The model under review builds one solid part; all positions refer to its coordinate system, in mm. A direction names the side the tool comes from. Coordinates: 2 decimals unless noted, no trailing zeros. Loops run counter-clockwise (first coordinate to the right, second up) from the corner with the lowest first, then second, coordinate; pieces in that order, holes last. Notation, with made-up numbers: M 24.5,-19.75 L 80.5,-19.75 A17 ccw 80.5,-6.75 Z; hole C -32.75,34.5 d6. An arc over 180 degrees is marked long. Return JSON: item names as keys, results as strings.
```python
from build123d import *

# Parameters (mm, degrees)
SKETCH1_R           = 2.542419914
BOSS_EXTRUDE1_DEPTH = 3.999992


with BuildPart() as part:
    # Sketch1 → Boss-Extrude1 (new body)
    with BuildSketch(Plane(origin=(0, 0, 0), x_dir=(1, 0, 0), z_dir=(0, 1, 0))):
        with BuildLine():
            Line((-7.927115113, 2.735422797), (-7.212976361, 2.491621041))
            ThreePointArc((-7.212976361, 2.491621041), (-6.913293064, 2.224424018), (-6.895509083, 1.823315483))
            ThreePointArc((-6.895509083, 1.823315483), (-6.953671189, 1.587130072), (-7.003745952, 1.349098778))
            ThreePointArc((-7.003745952, 1.349098778), (-7.193803236, 0.995428655), (-7.579741, 0.884720165))
            Line((-7.579741, 0.884720165), (-8.3289394, 0.974915565))
            ThreePointArc((-8.3289394, 0.974915565), (-9.212212433, 0.780173764), (-9.9866958, 0.3129788))
            Line((-9.9866958, 0.3129788), (-9.9866958, -0.3129788))
            ThreePointArc((-9.9866958, -0.3129788), (-9.212212433, -0.780173764), (-8.3289394, -0.974915565))
            Line((-8.3289394, -0.974915565), (-7.579741, -0.884720165))
            ThreePointArc((-7.579741, -0.884720165), (-7.193803236, -0.995428655), (-7.003745952, -1.349098778))
            ThreePointArc((-7.003745952, -1.349098778), (-6.953671189, -1.587130072), (-6.895509083, -1.823315483))
            ThreePointArc((-6.895509083, -1.823315483), (-6.913293064, -2.224424018), (-7.212976361, -2.491621041))
            Line((-7.212976361, -2.491621041), (-7.927115113, -2.735422797))
            ThreePointArc((-7.927115113, -2.735422797), (-8.638421316, -3.294116903), (-9.133498421, -4.05108076))
            Line((-9.133498421, -4.05108076), (-8.861905597, -4.61504907))
            ThreePointArc((-8.861905597, -4.61504907), (-7.961411897, -4.699941449), (-7.081115091, -4.492159943))
            Line((-7.081115091, -4.492159943), (-6.445244975, -4.085831692))
            ThreePointArc((-6.445244975, -4.085831692), (-6.049492451, -4.018124475), (-5.724805039, -4.25430748))
            ThreePointArc((-5.724805039, -4.25430748), (-5.576411329, -4.44703964), (-5.421532073, -4.63459975))
            ThreePointArc((-5.421532073, -4.63459975), (-5.263520415, -5.003702234), (-5.417593292, -5.374466142))
            Line((-5.417593292, -5.374466142), (-5.955228458, -5.903977126))
            ThreePointArc((-5.955228458, -5.903977126), (-6.353684915, -6.715967318), (-6.471299665, -7.612774092))
            Line((-6.471299665, -7.612774092), (-5.981906306, -8.003052272))
            ThreePointArc((-5.981906306, -8.003052272), (-5.133756094, -7.688828089), (-4.430789095, -7.119676951))
            Line((-4.430789095, -7.119676951), (-4.034189136, -6.477694143))
            ThreePointArc((-4.034189136, -6.477694143), (-3.707005493, -6.244981464), (-3.311996278, -6.31689841))
            ThreePointArc((-3.311996278, -6.31689841), (-3.094674815, -6.426158468), (-2.873754145, -6.527944698))
            ThreePointArc((-2.873754145, -6.527944698), (-2.571242995, -6.791935856), (-2.54918943, -7.192832311))
            Line((-2.54918943, -7.192832311), (-2.80383577, -7.903176378))
            ThreePointArc((-2.80383577, -7.903176378), (-2.810523293, -8.807638039), (-2.527380645, -9.666664151))
            Line((-2.527380645, -9.666664151), (-1.917117109, -9.805952821))
            ThreePointArc((-1.917117109, -9.805952821), (-1.289296936, -9.154848028), (-0.902890978, -8.337054622))
            Line((-0.902890978, -8.337054622), (-0.824112663, -7.586569825))
            ThreePointArc((-0.824112663, -7.586569825), (-0.630300635, -7.234943284), (-0.243206036, -7.128350138))
            ThreePointArc((-0.243206036, -7.128350138), (0, -7.1324978), (0.243206036, -7.128350138))
            ThreePointArc((0.243206036, -7.128350138), (0.630300635, -7.234943284), (0.824112663, -7.586569825))
            Line((0.824112663, -7.586569825), (0.902890978, -8.337054622))
            ThreePointArc((0.902890978, -8.337054622), (1.289296936, -9.154848028), (1.917117109, -9.805952821))
            Line((1.917117109, -9.805952821), (2.527380645, -9.666664151))
            ThreePointArc((2.527380645, -9.666664151), (2.810523293, -8.807638039), (2.80383577, -7.903176378))
            Line((2.80383577, -7.903176378), (2.54918943, -7.192832311))
            ThreePointArc((2.54918943, -7.192832311), (2.571242995, -6.791935856), (2.873754145, -6.527944698))
            ThreePointArc((2.873754145, -6.527944698), (3.094674815, -6.426158468), (3.311996278, -6.31689841))
            ThreePointArc((3.311996278, -6.31689841), (3.707005493, -6.244981464), (4.034189136, -6.477694143))
            Line((4.034189136, -6.477694143), (4.430789095, -7.119676951))
            ThreePointArc((4.430789095, -7.119676951), (5.133756094, -7.688828089), (5.981906306, -8.003052272))
            Line((5.981906306, -8.003052272), (6.471299665, -7.612774092))
            ThreePointArc((6.471299665, -7.612774092), (6.353684915, -6.715967318), (5.955228458, -5.903977126))
            Line((5.955228458, -5.903977126), (5.417593292, -5.374466142))
            ThreePointArc((5.417593292, -5.374466142), (5.263520415, -5.003702234), (5.421532073, -4.63459975))
            ThreePointArc((5.421532073, -4.63459975), (5.576411329, -4.44703964), (5.724805039, -4.25430748))
            ThreePointArc((5.724805039, -4.25430748), (6.049492451, -4.018124475), (6.445244975, -4.085831692))
            Line((6.445244975, -4.085831692), (7.081115091, -4.492159943))
            ThreePointArc((7.081115091, -4.492159943), (7.961411897, -4.699941449), (8.861905597, -4.61504907))
            Line((8.861905597, -4.61504907), (9.133498421, -4.05108076))
            ThreePointArc((9.133498421, -4.05108076), (8.638421316, -3.294116903), (7.927115113, -2.735422797))
            Line((7.927115113, -2.735422797), (7.212976361, -2.491621041))
            ThreePointArc((7.212976361, -2.491621041), (6.913293064, -2.224424018), (6.895509083, -1.823315483))
            ThreePointArc((6.895509083, -1.823315483), (6.953671189, -1.587130072), (7.003745952, -1.349098778))
            ThreePointArc((7.003745952, -1.349098778), (7.193803236, -0.995428655), (7.579741, -0.884720165))
            Line((7.579741, -0.884720165), (8.3289394, -0.974915565))
            ThreePointArc((8.3289394, -0.974915565), (9.212212433, -0.780173764), (9.9866958, -0.3129788))
            Line((9.9866958, -0.3129788), (9.9866958, 0.3129788))
            ThreePointArc((9.9866958, 0.3129788), (9.212212433, 0.780173764), (8.3289394, 0.974915565))
            Line((8.3289394, 0.974915565), (7.579741, 0.884720165))
            ThreePointArc((7.579741, 0.884720165), (7.193803236, 0.995428655), (7.003745952, 1.349098778))
            ThreePointArc((7.003745952, 1.349098778), (6.953671189, 1.587130072), (6.895509083, 1.823315483))
            ThreePointArc((6.895509083, 1.823315483), (6.913293064, 2.224424018), (7.212976361, 2.491621041))
            Line((7.212976361, 2.491621041), (7.927115113, 2.735422797))
            ThreePointArc((7.927115113, 2.735422797), (8.638421316, 3.294116903), (9.133498421, 4.05108076))
            Line((9.133498421, 4.05108076), (8.861905597, 4.61504907))
            ThreePointArc((8.861905597, 4.61504907), (7.961411897, 4.699941449), (7.081115091, 4.492159943))
            Line((7.081115091, 4.492159943), (6.445244975, 4.085831692))
            ThreePointArc((6.445244975, 4.085831692), (6.049492451, 4.018124475), (5.724805039, 4.25430748))
            ThreePointArc((5.724805039, 4.25430748), (5.576411329, 4.44703964), (5.421532073, 4.63459975))
            ThreePointArc((5.421532073, 4.63459975), (5.263520415, 5.003702234), (5.417593292, 5.374466142))
            Line((5.417593292, 5.374466142), (5.955228458, 5.903977126))
            ThreePointArc((5.955228458, 5.903977126), (6.353684915, 6.715967318), (6.471299665, 7.612774092))
            Line((6.471299665, 7.612774092), (5.981906306, 8.003052272))
            ThreePointArc((5.981906306, 8.003052272), (5.133756094, 7.688828089), (4.430789095, 7.119676951))
            Line((4.430789095, 7.119676951), (4.034189136, 6.477694143))
            ThreePointArc((4.034189136, 6.477694143), (3.707005493, 6.244981464), (3.311996278, 6.31689841))
            ThreePointArc((3.311996278, 6.31689841), (3.094674815, 6.426158468), (2.873754145, 6.527944698))
            ThreePointArc((2.873754145, 6.527944698), (2.571242995, 6.791935856), (2.54918943, 7.192832311))
            Line((2.54918943, 7.192832311), (2.80383577, 7.903176378))
            ThreePointArc((2.80383577, 7.903176378), (2.810523293, 8.807638039), (2.527380645, 9.666664151))
            Line((2.527380645, 9.666664151), (1.917117109, 9.805952821))
            ThreePointArc((1.917117109, 9.805952821), (1.289296936, 9.154848028), (0.902890978, 8.337054622))
            Line((0.902890978, 8.337054622), (0.824112663, 7.586569825))
            ThreePointArc((0.824112663, 7.586569825), (0.630300635, 7.234943284), (0.243206036, 7.128350138))
            ThreePointArc((0.243206036, 7.128350138), (0, 7.1324978), (-0.243206036, 7.128350138))
            ThreePointArc((-0.243206036, 7.128350138), (-0.630300635, 7.234943284), (-0.824112663, 7.586569825))
            Line((-0.824112663, 7.586569825), (-0.902890978, 8.337054622))
            ThreePointArc((-0.902890978, 8.337054622), (-1.289296936, 9.154848028), (-1.917117109, 9.805952821))
            Line((-1.917117109, 9.805952821), (-2.527380645, 9.666664151))
            ThreePointArc((-2.527380645, 9.666664151), (-2.810523293, 8.807638039), (-2.80383577, 7.903176378))
            Line((-2.80383577, 7.903176378), (-2.54918943, 7.192832311))
            ThreePointArc((-2.54918943, 7.192832311), (-2.571242995, 6.791935856), (-2.873754145, 6.527944698))
            ThreePointArc((-2.873754145, 6.527944698), (-3.094674815, 6.426158468), (-3.311996278, 6.31689841))
            ThreePointArc((-3.311996278, 6.31689841), (-3.707005493, 6.244981464), (-4.034189136, 6.477694143))
            Line((-4.034189136, 6.477694143), (-4.430789095, 7.119676951))
            ThreePointArc((-4.430789095, 7.119676951), (-5.133756094, 7.688828089), (-5.981906306, 8.003052272))
            Line((-5.981906306, 8.003052272), (-6.471299665, 7.612774092))
            ThreePointArc((-6.471299665, 7.612774092), (-6.353684915, 6.715967318), (-5.955228458, 5.903977126))
            Line((-5.955228458, 5.903977126), (-5.417593292, 5.374466142))
            ThreePointArc((-5.417593292, 5.374466142), (-5.263520415, 5.003702234), (-5.421532073, 4.63459975))
            ThreePointArc((-5.421532073, 4.63459975), (-5.576411329, 4.44703964), (-5.724805039, 4.25430748))
            ThreePointArc((-5.724805039, 4.25430748), (-6.049492451, 4.018124475), (-6.445244975, 4.085831692))
            Line((-6.445244975, 4.085831692), (-7.081115091, 4.492159943))
            ThreePointArc((-7.081115091, 4.492159943), (-7.961411897, 4.699941449), (-8.861905597, 4.61504907))
            Line((-8.861905597, 4.61504907), (-9.133498421, 4.05108076))
            ThreePointArc((-9.133498421, 4.05108076), (-8.638421316, 3.294116903), (-7.927115113, 2.735422797))
        make_face()
        with Locations(Location((0, 0, 0), (0, 0, 270))):
            Circle(SKETCH1_R, mode=Mode.SUBTRACT)
    extrude(amount=BOSS_EXTRUDE1_DEPTH)


solid = part.part
```
1. Add section B-B on z = 0. Give the boundary of the cut face in (x, y).
Check values:
{"outline": "M -9.99,0 L -2.54,0 L -2.54,4 L -9.99,4 Z; M 2.54,0 L 9.99,0 L 9.99,4 L 2.54,4 Z"}
2. Insertion check: pin 1 Ø2 at (x, y) = (-4, 1) entering from +Z; pin 2 Ø1 at (y, z) = (2, 7) entering from -X. Each pin has a flat end and moves straight along its axis. Give the tip position at first contact, or say it passes through.
Check values:
{"pin 1": "z = 7.61", "pin 2": "x = -6.47"}
3. Machinability: for faces 4 (the face through (-9.224, 1.972, 0.775)), 5 (the face through (6.357, 1.972, 6.728)), 6 (the face through (-5.145, 1.972, 7.695)), 7 (the face through (5.145, 1.972, -7.695)), which of the approach directions +Z, -Z, +X, -X, +Y, -Y give a long, thin tool a straight path to every point of the face, cutting with its end or side? Answer none if there is none.
Check values:
{"face 4": "-X, +Y, -Y", "face 5": "+X, +Y, -Y", "face 6": "+Z, +Y, -Y", "face 7": "-Z, +Y, -Y"}
4. Add section C-C on z = 5. Give the boundary of the cut face in (x, y).
Check values:
{"outline": "M -5.26,0 L 5.26,0 L 5.26,4 L -5.26,4 Z"}
5. Add section A-A on x = 0. Give the boundary of the cut face in (y, z), plus the area to 3 significant figures.
Check values:
{"outline": "M 0,-7.13 L 4,-7.13 L 4,-2.54 L 0,-2.54 Z; M 0,2.54 L 4,2.54 L 4,7.13 L 0,7.13 Z", "area": "36.7 mm²"}
6. The part is to be moulded in two halves that separate along X. For faces 1 (the face through (7.97, 1.97, -4.7)), 2 (the face through (-8.63, 1.972, 3.285)), 3 (the face through (8.63, 1.972, -3.285)), say which applies: released by +X, released by -X, zero draft, split by the parting line, or undercut.
Check values:
{"face 1": "undercut", "face 2": "released by -X", "face 3": "released by +X"}
7. Add section D-D on z = 3. Give the boundary of the cut face in (x, y).
Check values:
{"outline": "M -8.32,0 L 8.32,0 L 8.32,4 L -8.32,4 Z"}
8. To check wall thickness, follow line 1 (Z direction, x = 9, y = 1.85); line 2 (X direction, y = 3.15, z = -6.5); line 3 (X direction, y = 3.25, z = 0). State the ranges of each line that lie inside material, in increasing order.
Check values:
{"line 1": "-4.33 to -3.79, -0.86 to 0.86, 3.79 to 4.33", "line 2": "-6.28 to -4.05, -2.94 to 2.94, 4.05 to 6.28", "line 3": "-9.99 to -2.54, 2.54 to 9.99"}
